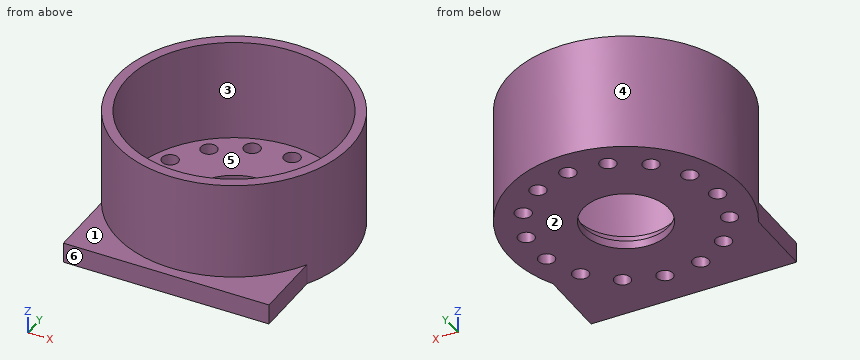
Autodesk Inventor part; units mm, degrees
ref_plane "YZ Plane" through (0, 0, 0) normal (1, 0, 0) x (0, 1, 0)
ref_plane "XZ Plane" through (0, 0, 0) normal (0, 1, 0) x (-1, 0, 0)
ref_plane "XY Plane" through (0, 0, 0) normal (0, 0, 1) x (1, 0, 0)
sketch "Sketch1" plane through (0, 0, 0) normal (0, 0, 1) x (1, 0, 0)
  circle A0 centre (0, 0) radius 52.5
  circle A1 centre (0, 0) radius 57.5
  circle A2 centre (0, 0) radius 23.6
  circle A3 centre (0, 0) radius 21.1
  circle A4 centre (0, 0) radius 45 construction
  line L0 (50.4975, -27.5) -> (50.4975, -62.5)
  line L1 (-50.4975, -27.5) -> (-50.4975, -62.5)
  line L2 (50.4975, -62.5) -> (-50.4975, -62.5)
  line L3 (20.0155, -57.5) -> (-14.9845, -57.5) construction
  circle A5 centre (-45, 0) radius 4
  dimension "d11" = 90
  dimension "d0" = 105
  dimension "d1" = 5
  dimension "d2" = 47.2
  dimension "d3" = 2.5
  dimension "d17" = 35
  dimension "d18" = 35
  dimension "d19" = 5
  dimension "d22" = 8
extrude "Extrusion1" add sketch "Sketch1" along normal blind 4 contours A2
extrude "Extrusion2" add sketch "Sketch1" along normal blind 8 contours A0 | A5
extrude "Extrusion3" add sketch "Sketch1" along normal blind 58 contours A1
extrude "Extrusion4" cut sketch "Sketch1" along normal blind 15 contours A5
extrude "Extrusion5" add sketch "Sketch1" along normal blind 10 contours A1 L0 L2 L1
pattern_circular "Circular Pattern2" count 15 over 360 about axis through (0, 0, 0) along (0, 0, 1) of "Extrusion4"
properties part number "Main Housing"
CAD build for the part. Positions are in the model's coordinates, mm. Face numbers are marked on the shaded views. A direction names the side the tool comes from. Give positions to 0.01 mm unless a question says otherwise; leave off trailing zeros. Loops run counter-clockwise (first coordinate to the right, second up) from the corner with the lowest first, then second, coordinate; pieces in that order, holes last. Notation, with made-up numbers: (51, 30.5) -> (71, 30.5) arc R25 cw to (71, 52.5) -> close; hole circle Ø6 at (53, 26.5). An arc over 180 degrees is marked (long way). Use a Markdown table: item, result.
1. Slice it at D-D (x = 35.5). List the corners of the cut face in (y, z), plus the area to 3 significant figures.
Check result:
| item | result |
|---|---|
| outline | (-62.5, 0) -> (-30.35, 0) -> (-30.35, 8) -> (-38.68, 8) -> (-38.68, 58) -> (-45.23, 58) -> (-45.23, 10) -> (-62.5, 10) -> close; (-22.55, 0) -> (22.55, 0) -> (22.55, 8) -> (-22.55, 8) -> close; (30.35, 0) -> (45.23, 0) -> (45.23, 58) -> (38.68, 58) -> (38.68, 8) -> (30.35, 8) -> close |
| area | 1,430 mm^2 |
2. Slice it at C-C (z = 32). List the corners of the cut face in (x, y).
Check result:
| item | result |
|---|---|
| outline | circle Ø115 at (0, 0); hole circle Ø105 at (0, 0) |
3. Which spindle directions (+Z, -Z, +X, -X, +Y, -Y) get a long thin tool onto all of the face, cutting with end or side? Do the marked faces 1, 2 and 3. Say none if no direction does.
Check result:
| item | result |
|---|---|
| face 1 | +Z, -Y |
| face 2 | -Z, +X, -X, +Y, -Y |
| face 3 | +Z |
4. Slice it at B-B (x = 13). List the corners of the cut face in (y, z).
Check result:
| item | result |
|---|---|
| outline | (-62.5, 0) -> (-16.62, 0) -> (-16.62, 4) -> (-19.7, 4) -> (-19.7, 8) -> (-50.87, 8) -> (-50.87, 58) -> (-56.01, 58) -> (-56.01, 10) -> (-62.5, 10) -> close; (16.62, 0) -> (56.01, 0) -> (56.01, 58) -> (50.87, 58) -> (50.87, 8) -> (19.7, 8) -> (19.7, 4) -> (16.62, 4) -> close |
5. Wall check: L1, parallel to X at y = -15.5, z = 3; L2, parallel to Z at x = 41, y = -17; L3, parallel to Y at x = -46.5, z = 27. Give the ranges that are in metal, low to high. Write a range as [from, to].
Check result:
| item | result |
|---|---|
| L1 | x = [-55.37, -43.96], [-38.26, -14.32], [14.32, 55.37] |
| L2 | z = [0, 8] |
| L3 | y = [-33.82, -24.37], [24.37, 33.82] |
6. Flat gauge pins, fed straight in: pin 1 (5 mm diameter, centred on x = -35.5, y = 30, fed in from -Z); pin 2 (8 mm diameter, centred on y = -48.5, z = 2.5, fed in from +X); pin 3 (6.5 mm diameter, centred on x = -13.91, y = 42.8, fed in from -Z); pin 4 (1.5 mm diameter, centred on x = -1.5, z = 12, fed in from +Y). Where does each tip first touch, or does it go through?
Check result:
| item | result |
|---|---|
| pin 1 | stops at z = 0 |
| pin 2 | stops at x = 50.5 |
| pin 3 | passes through |
| pin 4 | stops at y = 57.5 |
7. Slice it at A-A (y = 0). List the corners of the cut face in (x, z), plus the area to 3 significant figures.
Check result:
| item | result |
|---|---|
| outline | (-57.5, 0) -> (-49, 0) -> (-49, 8) -> (-52.5, 8) -> (-52.5, 58) -> (-57.5, 58) -> close; (-41, 0) -> (-21.1, 0) -> (-21.1, 4) -> (-23.6, 4) -> (-23.6, 8) -> (-41, 8) -> close; (21.1, 0) -> (57.5, 0) -> (57.5, 58) -> (52.5, 58) -> (52.5, 8) -> (23.6, 8) -> (23.6, 4) -> (21.1, 4) -> close |
| area | 998 mm^2 |
8. Mould opens along X. For the marked faces 4, 5 and 6 say: pulls with the +X half, pulls with the -X half, needs draft (parallel to the pull), parting line crosses it, or undercut.
Check result:
| item | result |
|---|---|
| face 4 | parting line crosses it |
| face 5 | undercut |
| face 6 | needs draft |
